Here's how the part is built. I have some questions about the finished solid (model axes, mm). A direction names the side the tool comes from. Round coordinates to 2 decimals unless told otherwise and drop trailing zeros. Write each loop counter-clockwise with the first axis right and the second up, starting at its lowest first coordinate (ties: lowest second). Pieces come first, ordered by that corner, then holes. Notation, with made-up numbers: (-35.75, 54.5) - (-21.75, 54.5) arc R15 cw to (-21.75, 67.5) - close; hole circle Ø7 at (-5, 34). An arc over 180 degrees is marked (long way). One line per question, with ' | ' between items. Start each with the question number.
(1) Imagine slicing it at D-D (x = -52). Write out the boundary of the cut face in (y, z).
(2) Imagine slicing it at A-A (x = 0). Write out the boundary of the cut face in (y, z) (1 decimal), plus the area to 3 significant figures.
(3) Thinking about a two-plate mould opening in X: for faces 1 (the cylindrical face through (-57.56, 3.83, -33.65)), 2 (the cylindrical face through (57.925, 3.828, -33.02)), 3 (the flat face through (34, 8.89, 53)), 4 (the cylindrical face through (-13.42, 4.51, 60.44)), which applies, pulls with the +X half, pulls with the -X half, needs draft (parallel to the pull), parting line crosses it, or undercut?
(4) If I drill on L1, parallel to X at y = 7, z = 0 (1 decimal); L2, parallel to Z at x = 0, y = 2.75 (1 decimal), over which ranges is the centre line in solid material (lowest first)?
(5) For faces 5 (the flat face through (4, 2.54, 65)), 6 (the cylindrical face through (-29.59, 4.38, 56.9)), 7 (the flat face through (55.3, 5.08, -32.9)), 8 (the flat face through (0.9, 5.08, 64.4)), which set-ups out of +Z, -Z, +X, -X, +Y, -Y let a thin tool reach every point of the face, with its end or its side?
(6) Imagine slicing it at B-B (z = 0). Write out the boundary of the cut face in (x, y) (1 decimal).
(7) Will these pins go through, and if not, where does the flat tip stop? pin 1 (5 mm diameter, centred on x = -5.5, y = 3, fed in from +Z); pin 2 (5 mm diameter, centred on y = 4, z = 10, fed in from -X); pin 3 (3 mm diameter, centred on x = -10, y = 5.5, fed in from +Z).
(8) Imagine slicing it at C-C (y = 7.5). Write out the boundary of the cut face in (x, z) (1 decimal).
Autodesk Inventor part; units mm, degrees
ref_plane "YZ Plane" through (0, 0, 0) normal (1, 0, 0) x (0, 1, 0)
ref_plane "XZ Plane" through (0, 0, 0) normal (0, 1, 0) x (-1, 0, 0)
ref_plane "XY Plane" through (0, 0, 0) normal (0, 0, 1) x (1, 0, 0)
sketch "Sketch1" plane through (0, 0, 0) normal (0, 1, 0) x (-1, 0, 0)
  circle A0 centre (0, 0) radius 64.135
  dimension "d0" = 128.27
extrude "Extrusion1" add sketch "Sketch1" along normal blind 8.89
sketch "Sketch2" plane through (0, 8.89, 0) normal (0, 1, 0) x (1, 0, 0)
  circle A0 centre (0, 0) radius 61.9125
  dimension "d3" = 123.825
extrude "Extrusion2" cut sketch "Sketch2" against normal through all
sketch "Sketch4" plane through (0, 0, 0) normal (1, 0, 0) x (0, 1, 0)
  line L0 (0, 64.135) -> (8.89, 64.135)
  line L1 (0, 64.135) -> (2.54, 64.135)
  line L2 (2.54, 64.135) -> (2.54, 66.675)
  line L3 (2.54, 66.675) -> (5.08, 66.675)
  line L4 (5.08, 66.675) -> (5.08, 64.135)
  line L5 (5.08, 64.135) -> (2.54, 64.135)
  line L6 (-1.778, 0) -> (10.668, 0)
  point P0 (0, 0)
  dimension "d17" = 2.54
  dimension "d18" = 2.54
  dimension "d19" = 2.54
revolve "Revolution1" add sketch "Sketch4" angle 45 mid plane about axis through (0, -10, 0) along (0, 1, 0)
sketch "Sketch6" plane through (-25.5154, 2.54, 61.5997) normal (-0.9238795, 0, -0.3826834) x (-0.3826834, 0, 0.9238795)
  line L0 (-2.54, 0) -> (-2.54, 2.54)
  line L1 (-2.54, 0) -> (0, 0)
  line L2 (0, 0) -> (0, -2.54)
  line L3 (0, -2.54) -> (-2.54, -2.54)
  line L4 (-2.54, -2.54) -> (-2.54, 0)
  line L5 (-66.675, -4.318) -> (-66.675, 8.128)
  point P0 (-66.675, -2.54)
  dimension "d21" = 2.54
  dimension "d22" = 2.54
revolve "Revolution2" add sketch "Sketch6" angle 5 about axis through (0, -10, 0) along (0, 1, 0)
fillet "Fillet3" radius 0.762 1 edges at (-19.6677, 2.54, 62.3779)
pattern_circular "Circular Pattern1" count 3 over 360 about axis through (0, -10, 0) along (0, 1, 0) of "Revolution1", "Revolution2", "Fillet3"
properties part number "bottom_thread"
Check sheet entries:
1) outline: (0, -37.54) - (2.54, -37.54) - (2.54, -41.73) - (5.08, -41.73) - (5.08, -37.54) - (8.89, -37.54) - (8.89, -33.6) - (0, -33.6) - close; (0, 33.6) - (8.89, 33.6) - (8.89, 37.54) - (0, 37.54) - close
2) outline: (0, -64.1) - (8.9, -64.1) - (8.9, -61.9) - (0, -61.9) - close; (0, 61.9) - (8.9, 61.9) - (8.9, 64.1) - (5.1, 64.1) - (5.1, 66.7) - (2.5, 66.7) - (2.5, 64.1) - (0, 64.1) - close | area: 46.0 mm^2
3) face 1: pulls with the -X half | face 2: pulls with the +X half | face 3: needs draft | face 4: undercut
4) L1: -64.1 to -61.9, 61.9 to 64.1 | L2: -64.1 to -61.9, 61.9 to 66.7
5) face 5: +Z, -Y | face 6: none | face 7: -Z, +X, +Y | face 8: +Z, +Y
6) outline: (-64.1, 0) - (-61.9, 0) - (-61.9, 8.9) - (-64.1, 8.9) - close; (61.9, 0) - (64.1, 0) - (64.1, 8.9) - (61.9, 8.9) - close
7) pin 1: z = 66.61 | pin 2: x = -63.69 | pin 3: z = 66.12
8) outline: circle Ø128.3 at (0, 0); hole circle Ø123.8 at (0, 0)
